```python
from build123d import *

# Parameters (mm, degrees)
SKETCH2_R           = 75
BOSS_EXTRUDE1_DEPTH = 20
FILLET1_R           = 5
BOSS_EXTRUDE2_DEPTH = 5
CHAMFER14_SIZE      = 2.5
CHAMFER15_SIZE      = 2.5
FILLET4_R           = 5
FILLET5_R           = 5
SKETCH4_R           = 10
BOSS_EXTRUDE8_DEPTH = 2.5
SKETCH5_R           = 5
CUT_EXTRUDE1_DEPTH  = 10
CHAMFER24_SIZE      = 1.5


with BuildPart() as part:
    # Sketch2 → Boss-Extrude1 (new body)
    with BuildSketch(Plane(origin=(0, 0, 0), x_dir=(1, 0, 0), z_dir=(0, 1, 0))):
        with Locations(Location((0, 0, 0), (0, 0, 270))):
            Circle(SKETCH2_R)
    extrude(amount=BOSS_EXTRUDE1_DEPTH)

    # Fillet1
    fillet1_edges = [part.edges().sort_by_distance(p)[0] for p in [
        (0, 20, -75),
    ]]
    fillet(fillet1_edges, radius=FILLET1_R)

    # Sketch3 → Boss-Extrude2 (add, symmetric)
    with BuildSketch(Plane.XY):
        with BuildLine():
            Line((-35, 20), (30, 20))
            ThreePointArc((30, 20), (17.980206761, 58.849975441), (14.988260139, 99.406655245))
            ThreePointArc((14.988260139, 99.406655245), (5.736147111, 113.859892363), (-11.023885447, 110.172214589))
            ThreePointArc((-11.023885447, 110.172214589), (-34.173411443, 68.05385799), (-35, 20))
        make_face()
    extrude(amount=BOSS_EXTRUDE2_DEPTH, both=True)

    # Chamfer14
    chamfer14_edges = [part.edges().sort_by_distance(p)[0] for p in [
        (-34.173411443, 68.05385799, -5),
        (17.980206761, 58.849975441, -5),
        (5.736147111, 113.859892363, -5),
    ]]
    chamfer(chamfer14_edges, length=CHAMFER14_SIZE)

    # Chamfer15
    chamfer15_edges = [part.edges().sort_by_distance(p)[0] for p in [
        (-34.173411443, 68.05385799, 5),
        (17.980206761, 58.849975441, 5),
        (5.736147111, 113.859892363, 5),
    ]]
    chamfer(chamfer15_edges, length=CHAMFER15_SIZE)

    # Fillet4
    fillet4_edges = [part.edges().sort_by_distance(p)[0] for p in [
        (-2.579776455, 20, 5),
    ]]
    fillet(fillet4_edges, radius=FILLET4_R)

    # Fillet5
    fillet5_edges = [part.edges().sort_by_distance(p)[0] for p in [
        (-2.579776455, 20, -5),
    ]]
    fillet(fillet5_edges, radius=FILLET5_R)

    # Sketch4 → Boss-Extrude8 (add, symmetric)
    with BuildSketch(Plane.XY.offset(5)):
        with Locations(Location((0, 100, 0), (0, 0, 180))):
            Circle(SKETCH4_R)
    extrude(amount=BOSS_EXTRUDE8_DEPTH, both=True)

    # Sketch5 → Cut-Extrude1 (cut)
    with BuildSketch(Plane(origin=(0, 0, -5), x_dir=(-1, 0, 0), z_dir=(0, 0, -1))):
        with Locations((0, 100)):
            Circle(SKETCH5_R)
    extrude(amount=-CUT_EXTRUDE1_DEPTH, mode=Mode.SUBTRACT)

    # Chamfer24
    chamfer24_edges = [part.edges().sort_by_distance(p)[0] for p in [
        (10, 100, 7.5),
    ]]
    chamfer(chamfer24_edges, length=CHAMFER24_SIZE)


solid = part.part
```
Work out the finished part from the listing and answer in its coordinate system (mm). A direction names the side the tool comes from. Round coordinates to 2 decimals unless told otherwise and drop trailing zeros. Order: outer loops, then holes, each group sorted by start corner. A loop starts at its lowest first (then second) coordinate and runs counter-clockwise, first axis right, second up.
Q1. Find the intervals of material crossed by line 1 along Y through (x, z) = (0, 0); line 2 along Z through (x, y) = (-31, 37); line 3 along Y through (x, z) = (-0.5, 5.5), in increasing order.
Solution:
line 1: y = 0 to 95, 105 to 115
line 2: z = -5 to 5
line 3: y = 0 to 22.82, 90.01 to 109.99
Q2. The mould has two halves that part along Y. Classify faces 1 (the flat face through (-5, 60, 5)), 2 (the flat face through (-5, 60, -5)), 3 (the flat face through (1, 0, -1)), 4 (the cylindrical face through (-34, 68.7, 0)): pulls with the +Y half, pulls with the -Y half, needs draft (parallel to the pull), parting line crosses it, or undercut.
Solution:
face 1: undercut
face 2: needs draft
face 3: pulls with the -Y half
face 4: undercut
Q3. Given pin 1 Ø18 at (x, y) = (-9.5, 49.5) entering from +Z; pin 2 Ø11.5 at (x, y) = (0, 100) entering from -Z; pin 3 Ø4 at (x, z) = (13.5, 55) entering from +Y; pin 4 Ø5 at (y, z) = (52.5, -9.5) entering from +X, each flat-ended and moving along its own axis, determine where each tip first touches the part or whether it passes through.
Solution:
pin 1: stops at z = 5
pin 2: stops at z = -5
pin 3: stops at y = 20
pin 4: passes through
Q4. A cutting plane is placed at A-A, the plane x = 0. Determine the outline of the cut face in (y, z).
Solution:
outline: (0, -75) - (15, -75) arc R5 ccw to (20, -70) - (20, -10) arc R5 cw to (25, -5) - (95, -5) - (95, 5) - (105, 5) - (105, -5) - (112.5, -5) - (115, -2.5) - (115, 2.5) - (112.5, 5) - (110, 5) - (110, 6) - (108.5, 7.5) - (91.5, 7.5) - (90, 6) - (90, 5) - (25, 5) arc R5 cw to (20, 10) - (20, 70) arc R5 ccw to (15, 75) - (0, 75) - close
Q5. A cutting plane is placed at B-B, the plane z = 0. Determine the outline of the cut face in (x, y), then the cut area to 3 significant figures.
Solution:
outline: (-75, 0) - (75, 0) - (75, 15) arc R5 ccw to (70, 20) - (30, 20) arc R180 cw to (14.99, 99.41) arc R15 ccw to (-11.02, 110.17) arc R100 ccw to (-35, 20) - (-70, 20) arc R5 ccw to (-75, 15) - close; hole circle Ø10 at (0, 100)
area: 7,470 mm2
Q6. A tool of negligible diameter and unlimited length cuts with its end or side. For faces 5 (the cylindrical face through (1.08, 95.12, -0.07)), 6 (the cylindrical face through (1.302, 90.085, 5.507)), 7 (the cylindrical face through (-4, 21, 7)), from which of +Z, -Z, +X, -X, +Y, -Y can it reach the whole face along a straight path? Write none if from no direction.
Solution:
face 5: -Z
face 6: +Z
face 7: +Z, +X, -X
